For this review, take the finished solid that the model builds, in its own axes (mm). Round coordinates to 2 decimals unless told otherwise and drop trailing zeros. Write item = value, one per line. Start each with the question number.
from build123d import *

# Parameters (mm, degrees)
SKETCH1_W           = 434
SKETCH1_H           = 434
BOSS_EXTRUDE1_DEPTH = 5
SKETCH2_R           = 2.5
CUT_EXTRUDE1_DEPTH  = 5
SKETCH3_R           = 30
CUT_EXTRUDE2_DEPTH  = 5


with BuildPart() as part:
    # Sketch1 → Boss-Extrude1 (new body)
    with BuildSketch(Plane(origin=(0, 0, 0), x_dir=(1, 0, 0), z_dir=(0, 1, 0))):
        Rectangle(SKETCH1_W, SKETCH1_H)
    extrude(amount=BOSS_EXTRUDE1_DEPTH)

    # Sketch2 → Cut-Extrude1 (cut)
    with BuildSketch(Plane(origin=(0, 5, 0), x_dir=(1, 0, 0), z_dir=(0, 1, 0))):
        with Locations(Location((-207, 130, 0), (0, 0, 270))):
            Circle(SKETCH2_R)
        with Locations(Location((-207, 0, 0), (0, 0, 270))):
            Circle(SKETCH2_R)
        with Locations(Location((-207, -130, 0), (0, 0, 90))):
            Circle(SKETCH2_R)
        with Locations(Location((207, -130, 0), (0, 0, 270))):
            Circle(SKETCH2_R)
        with Locations(Location((207, 0, 0), (0, 0, 90))):
            Circle(SKETCH2_R)
        with Locations(Location((207, 130, 0), (0, 0, 90))):
            Circle(SKETCH2_R)
        with Locations(Location((130, 207, 0), (0, 0, 270))):
            Circle(SKETCH2_R)
        with Locations(Location((0, 207, 0), (0, 0, 270))):
            Circle(SKETCH2_R)
        with Locations(Location((-130, 207, 0), (0, 0, 90))):
            Circle(SKETCH2_R)
        with Locations(Location((-130, -207, 0), (0, 0, 270))):
            Circle(SKETCH2_R)
        with Locations(Location((0, -207, 0), (0, 0, 90))):
            Circle(SKETCH2_R)
        with Locations(Location((130, -207, 0), (0, 0, 90))):
            Circle(SKETCH2_R)
    extrude(amount=-CUT_EXTRUDE1_DEPTH, mode=Mode.SUBTRACT)

    # Sketch3 → Cut-Extrude2 (cut)
    with BuildSketch(Plane(origin=(0, 5, 0), x_dir=(1, 0, 0), z_dir=(0, 1, 0))):
        with Locations(Location((0, 0, 0), (0, 0, 270))):
            Circle(SKETCH3_R)
    extrude(amount=-CUT_EXTRUDE2_DEPTH, mode=Mode.SUBTRACT)


solid = part.part
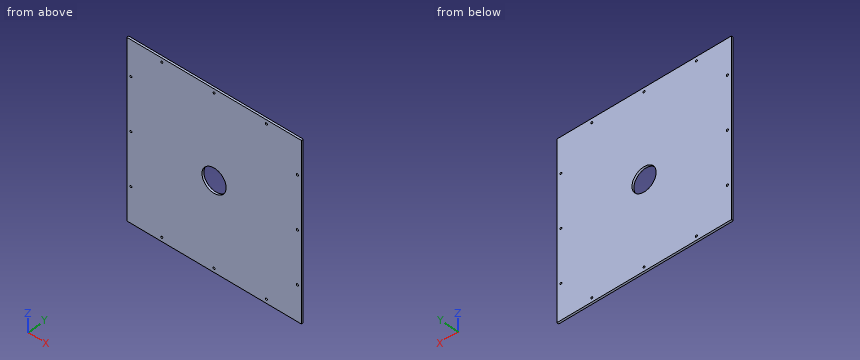
(1) For line 1 along X through (y, z) = (1.75, -130); line 2 along Z through (x, y) = (207, 1.75); line 3 along X through (y, z) = (3.3, 0), list the stretches that pass through material, from the lowest coordinate up.
(2) Insertion check: pin 1 (4 mm diameter, centred on x = 130, z = -207, fed in from -Y). The pin has a flat end and moves straight along its axis. Give the tip position at first contact, or say it passes through.
(3) We need section A-A, the plane y = 2.1. State how many separate pieces and enclosed holes the cut face has, then the cut area to 3 significant figures.
Values:
q1.line_1 = -217 to -209.5, -204.5 to 204.5, 209.5 to 217
q1.line_2 = -217 to -132.5, -127.5 to -2.5, 2.5 to 127.5, 132.5 to 217
q1.line_3 = -217 to -209.5, -204.5 to -30, 30 to 204.5, 209.5 to 217
q2.pin_1 = through
q3.separate_pieces = 1
q3.enclosed_holes = 13
q3.area = 185,000 mm²
